```python
from build123d import *

# Parameters (mm, degrees)
SKETCH038_W      = 36
SKETCH038_H      = 27.5
SKETCH038_W_2    = 30
SKETCH038_H_2    = 21.5
EXTRUDE026_DEPTH = 1
SKETCH039_R      = 4.8
SKETCH039_R_2    = 4
EXTRUDE027_DEPTH = 2.6
SKETCH037_W      = 64
SKETCH037_H      = 36
SKETCH037_R      = 4
SKETCH037_W_2    = 30
SKETCH037_H_2    = 21.5
EXTRUDE025_DEPTH = 3
CHAMFER_SIZE     = 2.4


with BuildPart() as basebevel001:
    # Sketch038 → Extrude026 (new body)
    with BuildSketch(Plane.XY):
        with Locations((34, 97.75)):
            Rectangle(SKETCH038_W, SKETCH038_H)
        with Locations((34, 97.75)):
            Rectangle(SKETCH038_W_2, SKETCH038_H_2, mode=Mode.SUBTRACT)
    extrude(amount=EXTRUDE026_DEPTH)


with BuildPart() as basebevel001_1:
    # Extrude026 placement: moved
    add(basebevel001.part.moved(Location((0, 0, 6.6))))


with BuildPart() as basebutton_t001:
    # Sketch039 → Extrude027 (new body)
    with BuildSketch(Plane.XY):
        with Locations((58.3, 97.8)):
            Circle(SKETCH039_R)
        with Locations((58.3, 97.8)):
            Circle(SKETCH039_R_2, mode=Mode.SUBTRACT)
    extrude(amount=EXTRUDE027_DEPTH)


with BuildPart() as basebutton_t001_1:
    # Extrude027 placement: moved
    add(basebutton_t001.part.moved(Location((0, 0, 5))))


with BuildPart() as obj1:
    # Sketch037 → Extrude025 (new body)
    with BuildSketch(Plane.XY):
        with Locations((34, 102)):
            Rectangle(SKETCH037_W, SKETCH037_H)
        with Locations((9.6, 98.3)):
            Circle(SKETCH037_R, mode=Mode.SUBTRACT)
        with Locations((58.3, 97.8)):
            Circle(SKETCH037_R, mode=Mode.SUBTRACT)
        with Locations((34, 97.75)):
            Rectangle(SKETCH037_W_2, SKETCH037_H_2, mode=Mode.SUBTRACT)
    extrude(amount=EXTRUDE025_DEPTH)


with BuildPart() as obj1_1:
    # Extrude025 placement: moved
    add(obj1.part.moved(Location((0, 0, 7.6))))

    # Fusion015: union basebevel001, basebutton_t001
    add(basebevel001_1.part)
    add(basebutton_t001_1.part)

    # Chamfer
    chamfer_edges = [obj1_1.edges().sort_by_distance(p)[0] for p in [
        (54.3, 97.8, 10.6),
        (5.6, 98.3, 10.6),
        (49, 97.75, 10.6),
        (19, 97.75, 10.6),
    ]]
    chamfer(chamfer_edges, length=CHAMFER_SIZE)


solid = obj1_1.part
```
Part model, mm, in its own coordinate system. A direction names the side the tool comes from. Round coordinates to 2 decimals unless told otherwise and drop trailing zeros. Order: outer loops, then holes, each group sorted by start corner. A loop starts at its lowest first (then second) coordinate and runs counter-clockwise, first axis right, second up. Notation, with made-up numbers: M 57.25,86 L 101.25,86 A21 cw 101.25,108 Z; hole C 41.5,4 d6. An arc over 180 degrees is marked long. Put each result on its own line as item: value. Start each with the question number.
1. Slice it at D-D on z = 5.7. List the corners of the cut face in (x, y), then the cut area to 3 significant figures.
2. Two-plate mould, pull along Y, no slides. Class faces 1 (the face through (34, 114, 7.6)), 2 (the face through (19, 98, 7)), 3 (the face through (11.446, 94.751, 7.896)), 4 (the face through (34, 120, 9)): +Y half, -Y half, draft (parallel to the pull), parting line (faces both ways), or undercut.
3. Slice it at C-C on y = 109.5. List the corners of the cut face in (x, z).
4. Slice it at A-A on x = 58.3. List the corners of the cut face in (y, z), then the cut area to 3 significant figures.
5. Slice it at B-B on z = 9.6. List the corners of the cut face in (x, y), then the cut area to 3 significant figures.
6. Tool access for faces 5 (the face through (34, 86, 6.6)), 6 (the face through (17.8, 97.6, 9.4)): list every direction of +Z, -Z, +X, -X, +Y, -Y with a clear straight run to the whole face (end or side of a thin tool).
7. Drop flat-ended pins along their axis: pin 1 (6.5 mm diameter, centred on x = 58.3, y = 97.8, fed in from -Z); pin 2 (0.8 mm diameter, centred on y = 93.5, z = 7, fed in from -X); pin 3 (1.5 mm diameter, centred on x = 54.5, z = 5.5, fed in from +Y); pin 4 (1.1 mm diameter, centred on x = 36, z = 7, fed in from +Y). Give the stop position or say it passes through.
8. Drill centre lines: probe 1 along Y at (x, z) = (58.3, 6.2); probe 2 along Y at (x, z) = (29.5, 8.25); probe 3 along X at (y, z) = (94.5, 9.4). Where is each one in solid material? Low to high. Write a range as [from, to].
Findings:
1. outline: C 58.3,97.8 d9.6; hole C 58.3,97.8 d8
1. area: 22.1 mm2
2. face 1: draft
2. face 2: undercut
2. face 3: undercut
2. face 4: +Y half
3. outline: M 2,7.6 L 16,7.6 L 16,6.6 L 52,6.6 L 52,7.6 L 66,7.6 L 66,10.6 L 2,10.6 Z
4. outline: M 84,7.6 L 93,7.6 L 93,5 L 93.8,5 L 93.8,8.2 L 91.4,10.6 L 84,10.6 Z; M 101.8,5 L 102.6,5 L 102.6,7.6 L 120,7.6 L 120,10.6 L 104.2,10.6 L 101.8,8.2 Z
4. area: 82.4 mm2
5. outline: M 2,84 L 66,84 L 66,120 L 2,120 Z; hole C 9.6,98.3 d10.8; hole M 17.6,87 L 50.4,87 L 50.4,108.5 L 17.6,108.5 Z; hole C 58.3,97.8 d10.8
5. area: 1,420 mm2
6. face 5: -Z, -X, +Y, -Y
6. face 6: +Z
7. pin 1: through
7. pin 2: x = 16
7. pin 3: y = 101.51
7. pin 4: y = 111.5
8. probe 1: [93, 93.8], [101.8, 102.6]
8. probe 2: [84, 87], [108.5, 120]
8. probe 3: [2, 6.05], [13.15, 17.8], [50.2, 54.28], [62.32, 66]
